Design review of the part built by this model. Coordinates are the model's own, in mm. A direction names the side the tool comes from. Give positions to 0.01 mm unless a question says otherwise; leave off trailing zeros. Loops run counter-clockwise (first coordinate to the right, second up) from the corner with the lowest first, then second, coordinate; pieces in that order, holes last. Notation, with made-up numbers: (11, 45.5) - (20, 45.5) arc R15 cw to (20, 56.5) - close; hole circle Ø8 at (3, 67). An arc over 180 degrees is marked (long way). Put each result on its own line as item: value. Start each with the question number.
```python
from build123d import *

# Parameters (mm, degrees)
SKETCH1_W           = 20
SKETCH1_H           = 6.5
BOSS_EXTRUDE1_DEPTH = 10.5
BOSS_EXTRUDE2_START = 5
BOSS_EXTRUDE2_DEPTH = 5
BOSS_EXTRUDE3_START = 2
BOSS_EXTRUDE3_DEPTH = 2
SKETCH7_W           = 12.2
SKETCH7_H           = 2
BOSS_EXTRUDE5_DEPTH = 3
FILLET2_R           = 2
CUT_EXTRUDE2_REACH  = 34.554
SKETCH8_R           = 1.6
CUT_EXTRUDE3_REACH  = 36.925
FILLET8_R           = 0.5
FILLET9_R           = 1
CUT_EXTRUDE4_REACH  = 36.411
SKETCH10_R          = 1.25


with BuildPart() as part:
    # Sketch1 → Boss-Extrude1 (new body)
    with BuildSketch(Plane(origin=(0, 0, 0), x_dir=(1, 0, 0), z_dir=(0, 1, 0))):
        with BuildLine():
            Line((0, 0), (0, 8.1))
            Line((0, 8.1), (12.2, 8.1))
            Line((12.2, 8.1), (12.2, 0))
            Line((12.2, 0), (27.7, 0))
            Line((27.7, 0), (27.7, 4.5))
            ThreePointArc((27.7, 4.5), (27.553553391, 4.853553391), (27.2, 5))
            Line((27.2, 5), (18.6, 5))
            ThreePointArc((18.6, 5), (18.246446609, 5.146446609), (18.1, 5.5))
            Line((18.1, 5.5), (18.1, 17.5))
            ThreePointArc((18.1, 17.5), (17.807106781, 18.207106781), (17.1, 18.5))
            Line((17.1, 18.5), (-4.9, 18.5))
            ThreePointArc((-4.9, 18.5), (-5.607106781, 18.207106781), (-5.9, 17.5))
            Line((-5.9, 17.5), (-5.9, 5.5))
            ThreePointArc((-5.9, 5.5), (-6.046446609, 5.146446609), (-6.4, 5))
            Line((-6.4, 5), (-15, 5))
            ThreePointArc((-15, 5), (-15.353553391, 4.853553391), (-15.5, 4.5))
            Line((-15.5, 4.5), (-15.5, 0))
            Line((-15.5, 0), (0, 0))
        make_face()
        with Locations((6.1, 13.35)):
            Rectangle(SKETCH1_W, SKETCH1_H, mode=Mode.SUBTRACT)
    extrude(amount=BOSS_EXTRUDE1_DEPTH)

    # Sketch5 → Boss-Extrude2 (add)
    with BuildSketch(Plane.XZ.offset(BOSS_EXTRUDE2_START)):
        with BuildLine():
            Line((0, -8.1), (-5.9, -8.1))
            Line((-5.9, -8.1), (-5.9, -17.5))
            ThreePointArc((-5.9, -17.5), (-5.607106781, -18.207106781), (-4.9, -18.5))
            Line((-4.9, -18.5), (17.1, -18.5))
            ThreePointArc((17.1, -18.5), (17.807106781, -18.207106781), (18.1, -17.5))
            Line((18.1, -17.5), (18.1, -8.1))
            Line((18.1, -8.1), (12.2, -8.1))
            Line((12.2, -8.1), (12.2, -10.1))
            Line((12.2, -10.1), (16.1, -10.1))
            Line((16.1, -10.1), (16.1, -16.6))
            Line((16.1, -16.6), (-3.9, -16.6))
            Line((-3.9, -16.6), (-3.9, -10.1))
            Line((-3.9, -10.1), (0, -10.1))
            Line((0, -10.1), (0, -8.1))
        make_face()
    extrude(amount=-BOSS_EXTRUDE2_DEPTH)

    # Sketch6 → Boss-Extrude3 (add)
    with BuildSketch(Plane.XZ.offset(5).offset(BOSS_EXTRUDE3_START)):
        with BuildLine():
            Line((-5.9, -8.1), (18.1, -8.1))
            Line((18.1, -8.1), (18.1, -17.5))
            ThreePointArc((18.1, -17.5), (17.807106781, -18.207106781), (17.1, -18.5))
            Line((17.1, -18.5), (-4.9, -18.5))
            ThreePointArc((-4.9, -18.5), (-5.607106781, -18.207106781), (-5.9, -17.5))
            Line((-5.9, -17.5), (-5.9, -8.1))
        make_face()
    extrude(amount=-BOSS_EXTRUDE3_DEPTH)

    # Sketch7 → Boss-Extrude5 (add)
    with BuildSketch(Plane.XY.offset(-8.1)):
        with Locations((6.1, 1)):
            Rectangle(SKETCH7_W, SKETCH7_H)
    extrude(amount=BOSS_EXTRUDE5_DEPTH)

    # Fillet2
    fillet2_edges = [part.edges().sort_by_distance(p)[0] for p in [
        (12.2, 1, -5.1),
        (0, 1, -5.1),
    ]]
    fillet(fillet2_edges, radius=FILLET2_R)

    # Sketch8 → Cut-Extrude2 (cut, up to next)
    with BuildSketch(Plane(origin=(0, 0, -5), x_dir=(-1, 0, 0), z_dir=(0, 0, -1)), mode=Mode.PRIVATE) as cut_extrude2_sk1:
        with Locations((-21.95, 5.25)):
            Circle(SKETCH8_R)
    cut_extrude2_tool1 = extrude(cut_extrude2_sk1.sketch, amount=-CUT_EXTRUDE2_REACH, mode=Mode.PRIVATE) & part.part
    # Sketch8 → Cut-Extrude2 (cut, up to next)
    with BuildSketch(Plane(origin=(0, 0, -5), x_dir=(-1, 0, 0), z_dir=(0, 0, -1)), mode=Mode.PRIVATE) as cut_extrude2_sk2:
        with Locations((9.75, 5.25)):
            Circle(SKETCH8_R)
    cut_extrude2_tool2 = extrude(cut_extrude2_sk2.sketch, amount=-CUT_EXTRUDE2_REACH, mode=Mode.PRIVATE) & part.part
    add(cut_extrude2_tool1.solids().sort_by_distance((21.95, 5.25, -5))[0], mode=Mode.SUBTRACT)
    add(cut_extrude2_tool2.solids().sort_by_distance((-9.75, 5.25, -5))[0], mode=Mode.SUBTRACT)

    # Sketch9 → Cut-Extrude3 (cut, up to next)
    with BuildSketch(Plane.XZ, mode=Mode.PRIVATE) as cut_extrude3_sk1:
        with BuildLine():
            Line((24.52766766, 0), (27.392231541, -4.961570184))
            ThreePointArc((27.392231541, -4.961570184), (27.616002266, -4.777384417), (27.7, -4.5))
            Line((27.7, -4.5), (27.7, 0))
            Line((27.7, 0), (24.52766766, 0))
        make_face()
    cut_extrude3_tool1 = extrude(cut_extrude3_sk1.sketch, amount=-CUT_EXTRUDE3_REACH, mode=Mode.PRIVATE) & part.part
    # Sketch9 → Cut-Extrude3 (cut, up to next)
    with BuildSketch(Plane.XZ, mode=Mode.PRIVATE) as cut_extrude3_sk2:
        with BuildLine():
            Line((-12.327667659, 0), (-15.5, 0))
            Line((-15.5, 0), (-15.5, -4.5))
            ThreePointArc((-15.5, -4.5), (-15.416002266, -4.777384417), (-15.19223154, -4.961570184))
            Line((-15.19223154, -4.961570184), (-12.327667659, 0))
        make_face()
    cut_extrude3_tool2 = extrude(cut_extrude3_sk2.sketch, amount=-CUT_EXTRUDE3_REACH, mode=Mode.PRIVATE) & part.part
    add(cut_extrude3_tool1.solids().sort_by_distance((26.628979, 0, -1.786116))[0], mode=Mode.SUBTRACT)
    add(cut_extrude3_tool2.solids().sort_by_distance((-14.428979, 0, -1.786116))[0], mode=Mode.SUBTRACT)

    # Fillet8
    fillet8_edges = [part.edges().sort_by_distance(p)[0] for p in [
        (-12.327667659, 5.25, 0),
    ]]
    fillet(fillet8_edges, radius=FILLET8_R)
    fillet8_2_edges = [part.edges().sort_by_distance(p)[0] for p in [
        (-15.19223154, 5.25, -4.961570184),
    ]]
    fillet(fillet8_2_edges, radius=FILLET8_R)
    fillet8_3_edges = [part.edges().sort_by_distance(p)[0] for p in [
        (27.392231541, 5.25, -4.961570184),
    ]]
    fillet(fillet8_3_edges, radius=FILLET8_R)
    fillet8_4_edges = [part.edges().sort_by_distance(p)[0] for p in [
        (24.52766766, 5.25, 0),
    ]]
    fillet(fillet8_4_edges, radius=FILLET8_R)

    # Fillet9
    fillet9_edges = [part.edges().sort_by_distance(p)[0] for p in [
        (-5.9, -7, -12.8),
        (18.1, -7, -12.8),
        (6.1, -7, -8.1),
        (-5.607106781, -7, -18.207106781),
        (6.1, -7, -18.5),
        (17.807106781, -7, -18.207106781),
    ]]
    fillet(fillet9_edges, radius=FILLET9_R)

    # Sketch10 → Cut-Extrude4 (cut, up to next)
    with BuildSketch(Plane(origin=(0, 0, -18.5), x_dir=(-1, 0, 0), z_dir=(0, 0, -1)), mode=Mode.PRIVATE) as cut_extrude4_sk1:
        with Locations((-11.25, 2.75)):
            Circle(SKETCH10_R)
    cut_extrude4_tool1 = extrude(cut_extrude4_sk1.sketch, amount=-CUT_EXTRUDE4_REACH, mode=Mode.PRIVATE) & part.part
    # Sketch10 → Cut-Extrude4 (cut, up to next)
    with BuildSketch(Plane(origin=(0, 0, -18.5), x_dir=(-1, 0, 0), z_dir=(0, 0, -1)), mode=Mode.PRIVATE) as cut_extrude4_sk2:
        with Locations((-1.9, 2.75)):
            Circle(SKETCH10_R)
    cut_extrude4_tool2 = extrude(cut_extrude4_sk2.sketch, amount=-CUT_EXTRUDE4_REACH, mode=Mode.PRIVATE) & part.part
    add(cut_extrude4_tool1.solids().sort_by_distance((11.25, 2.75, -18.5))[0], mode=Mode.SUBTRACT)
    add(cut_extrude4_tool2.solids().sort_by_distance((1.9, 2.75, -18.5))[0], mode=Mode.SUBTRACT)


solid = part.part
```
Item 1: Consider section D-D (x = 15). State the section outline as (y, z) points.
Item 2: For L1, parallel to Z at x = 11, y = 8; L2, parallel to X at y = 8.5, z = -13; L3, parallel to Z at x = 14, y = 9, list the stretches that pass through material, from the lowest coordinate up. Write a range as from..to.
Item 3: Consider section A-A (x = 21.95). State the section outline as (y, z) points.
Item 4: Consider section B-B (y = 5.25). Count the separate pieces of the cut face and the enclosed holes in it, plus the area to 3 significant figures.
Item 5: Consider section C-C (z = -11.75). State the section outline as (x, y) points.
Item 6: For P1, Ø1, axis at y = 1, z = -8, coming from the +X side; P2, Ø1, axis at x = 3.5, y = 3.5, coming from the +Z side; P3, Ø8.5, axis at x = -12, y = 4.5, coming from the -Z side, all flat-tipped, find the tip position at first contact; note any pin that passes through.
Item 7: Machinability: for faces 4 (the flat face through (0, -3, -9)), 5 (the flat face through (6, 1, -5.1)), 6 (the flat face through (12.2, 6, -4)), which of the approach directions +Z, -Z, +X, -X, +Y, -Y give a long, thin tool a straight path to every point of the face, cutting with its end or side? Answer none if there is none.
Item 8: Mouldability with a two-part tool opening along Y and no side actions: class faces 1 (the flat face through (6, -7, -13)), 2 (the flat face through (6, -5, -12)), 3 (the flat face through (16.1, 3, -13)) as pulls with the +Y half, pulls with the -Y half, needs draft (parallel to the pull), parting line crosses it, or undercut.
Geometry says:
1. outline: (-7, -17.5) arc R1 ccw to (-6, -18.5) - (10.5, -18.5) - (10.5, -16.6) - (-5, -16.6) - (-5, -10.1) - (10.5, -10.1) - (10.5, 0) - (0, 0) - (0, -8.1) - (-6, -8.1) arc R1 ccw to (-7, -9.1) - close
2. L1: z = -18.5..-16.6, -10.1..-8.1
2. L2: x = -5.9..-3.9, 16.1..18.1
2. L3: z = -18.5..-16.6, -10.1..0
3. outline: (0, -5) - (3.65, -5) - (3.65, 0) - (0, 0) - close; (6.85, -5) - (10.5, -5) - (10.5, 0) - (6.85, 0) - close
4. separate pieces: 3
4. enclosed holes: 1
4. area: 261 mm2
5. outline: (-5.9, -6) arc R1 ccw to (-4.9, -7) - (17.1, -7) arc R1 ccw to (18.1, -6) - (18.1, 10.5) - (16.1, 10.5) - (16.1, -5) - (-3.9, -5) - (-3.9, 10.5) - (-5.9, 10.5) - close
6. P1: stops at x = 18.1
6. P2: stops at z = -8.1
6. P3: stops at z = -5
7. face 4: +Z
7. face 5: +Z, +Y, -Y
7. face 6: +Z, +Y
8. face 1: pulls with the -Y half
8. face 2: undercut
8. face 3: needs draft
